Input: part model. Units: mm. Frame: model coordinates. Coordinates: 2 decimals unless noted, no trailing zeros. Loops run counter-clockwise (first coordinate to the right, second up) from the corner with the lowest first, then second, coordinate; pieces in that order, holes last. Notation, with made-up numbers: (49, 36.5) - (80, 36.5) arc R28 ccw to (80, 72.5) - close; hole circle Ø4 at (74.5, 38). An arc over 180 degrees is marked (long way). Write item = value, one per line. Start each with the question number.
from build123d import *

# Parameters (mm, degrees)
SKETCH1_R           = 4
EXTRUDE2_DEPTH      = 323.625
EXTRUDE2_DEPTH_BACK = 323.625
FILLET2_R           = 1
FILLET3_R           = 1


with BuildPart() as part:
    # Sketch1 → Extrude2 (new body, two sides)
    with BuildSketch(Plane.XY) as extrude2_sk:
        Circle(SKETCH1_R)
    extrude(amount=EXTRUDE2_DEPTH)
    extrude(extrude2_sk.sketch, amount=-EXTRUDE2_DEPTH_BACK)

    # Fillet2
    fillet2_edges = [part.edges().sort_by_distance(p)[0] for p in [
        (-4, 0, -323.625),
    ]]
    fillet(fillet2_edges, radius=FILLET2_R)

    # Fillet3
    fillet3_edges = [part.edges().sort_by_distance(p)[0] for p in [
        (-4, 0, 323.625),
    ]]
    fillet(fillet3_edges, radius=FILLET3_R)


solid = part.part
Item 1: Cut plane A-A on z = -212.5. Return loops of the section in (x, y), plus the area to 3 significant figures.
Item 2: Ray query, line 1 (Y direction, x = 0.25, z = 247); line 2 (Y direction, x = -2.5, z = 244); line 3 (X direction, y = 0.75, z = -170.5). Return the intervals inside material, ascending.
Item 3: Pin query (flat end, axial travel): pin 1 (3 mm diameter, centred on x = 3, z = 42, fed in from -Y); pin 2 (1.5 mm diameter, centred on y = 1, z = -168, fed in from +X); pin 3 (1 mm diameter, centred on y = -2, z = 169.5, fed in from +X). Return the tip coordinate at first contact, or that it passes through.
Recorded:
q1.outline = circle Ø8 at (0, 0)
q1.area = 50.3 mm²
q2.line_1 = -3.99 to 3.99
q2.line_2 = -3.12 to 3.12
q2.line_3 = -3.93 to 3.93
q3.pin_1 = -3.71
q3.pin_2 = 3.99
q3.pin_3 = 3.71
